The listing builds one solid part. Answer for the finished solid, in the listing's coordinates (mm). A direction names the side the tool comes from. Give positions to 0.01 mm unless a question says otherwise; leave off trailing zeros. Write each loop counter-clockwise with the first axis right and the second up, starting at its lowest first coordinate (ties: lowest second). Pieces come first, ordered by that corner, then holes. Notation, with made-up numbers: M -22.5,61.25 L 30.5,61.25 A27 cw 30.5,84.25 Z; hole C 16,-5.75 d5. An arc over 180 degrees is marked long. Answer as a JSON object with one key per item and string values.
```python
from build123d import *

# Parameters (mm, degrees)
SKETCH3_W           = 20
SKETCH3_H           = 15
BOSS_EXTRUDE1_DEPTH = 20
SKETCH5_R           = 5
CUT_EXTRUDE1_DEPTH  = 10
SKETCH6_R           = 5
CUT_EXTRUDE2_DEPTH  = 4


with BuildPart() as part:
    # Sketch3 → Boss-Extrude1 (new body)
    with BuildSketch(Plane(origin=(0, 0, 0), x_dir=(1, 0, 0), z_dir=(0, 1, 0))):
        Rectangle(SKETCH3_W, SKETCH3_H)
    extrude(amount=BOSS_EXTRUDE1_DEPTH)

    # Sketch5 → Cut-Extrude1 (cut)
    with BuildSketch(Plane(origin=(10, 0, 0), x_dir=(0, 0, -1), z_dir=(1, 0, 0))):
        with Locations((0, 10)):
            Circle(SKETCH5_R)
    extrude(amount=-CUT_EXTRUDE1_DEPTH, mode=Mode.SUBTRACT)

    # Sketch6 → Cut-Extrude2 (cut)
    with BuildSketch(Plane.ZY.offset(10)):
        with Locations((0, 10)):
            Circle(SKETCH6_R)
    extrude(amount=-CUT_EXTRUDE2_DEPTH, mode=Mode.SUBTRACT)


solid = part.part
```
1. A flat-ended cylindrical pin translates along its axis: pin 1 (6 mm diameter, centred on y = 10, z = 0, fed in from -X). Find the tip coordinate at first contact, or state that the pin passes through.
Verdict:
{"pin 1": "stops at x = -6"}
2. A cutting plane is placed at A-A, the plane y = 10. Give the vertices of the cut face in (x, z), plus the area to 3 significant figures.
Verdict:
{"outline": "M -10,-7.5 L 10,-7.5 L 10,-5 L 0,-5 L 0,5 L 10,5 L 10,7.5 L -10,7.5 L -10,5 L -6,5 L -6,-5 L -10,-5 Z", "area": "160 mm2"}
3. A cutting plane is placed at C-C, the plane x = 8. Give the vertices of the cut face in (y, z), plus the area to 3 significant figures.
Verdict:
{"outline": "M 0,-7.5 L 20,-7.5 L 20,7.5 L 0,7.5 Z; hole C 10,0 d10", "area": "221 mm2"}
4. For faces 5 (the flat face through (-6, 10, 0)), 6 (the flat face through (0, 10, 0)), 7 (the flat face through (-10, 8, 5)), determine the directions among +Z, -Z, +X, -X, +Y, -Y from which every point of the face is accessible in a straight line to the end or side of a thin tool.
Verdict:
{"face 5": "-X", "face 6": "+X", "face 7": "+Z, -Z, -X, +Y, -Y"}
5. The mould has two halves that part along Z. Classify faces 1 (the flat face through (0, 0, 0)), 2 (the flat face through (0, 10, -7.5)), 3 (the flat face through (0, 10, 7.5)), 4 (the cylindrical face through (5.07, 14.957, 0.651)): released by +Z, released by -Z, zero draft, split by the parting line, or undercut.
Verdict:
{"face 1": "zero draft", "face 2": "released by -Z", "face 3": "released by +Z", "face 4": "undercut"}
6. A cutting plane is placed at B-B, the plane z = 0. Give the vertices of the cut face in (x, y).
Verdict:
{"outline": "M -10,0 L 10,0 L 10,5 L 0,5 L 0,15 L 10,15 L 10,20 L -10,20 L -10,15 L -6,15 L -6,5 L -10,5 Z"}
7. Consider line 1 along Y through (x, z) = (6, 0); line 2 along Y through (x, z) = (-6.25, -4); line 3 along Z through (x, y) = (-6.25, 13.5). Determine where each line is inside the solid, lowest interval first.
Verdict:
{"line 1": "y = 0 to 5, 15 to 20", "line 2": "y = 0 to 7, 13 to 20", "line 3": "z = -7.5 to -3.57, 3.57 to 7.5"}
